from build123d import *

# Parameters (mm, degrees)
F10_DEPTH = 2
F11_DEPTH = 2
F12_DEPTH = 2
F13_DEPTH = 2
F14_W     = 8.485019207
F14_H     = 5.5162683129
F15_DEPTH = 25.4
F16_W     = 22.2342889756
F16_H     = 4.6487008221
F17_DEPTH = 25.4
F18_W     = 7.9449899495
F18_H     = 7.2886322159
F19_DEPTH = 25.4
F20_W     = 5.9225577861
F20_H     = 11.3939000294
F21_DEPTH = 25.4
F22_DEPTH = 25.4
F24_DEPTH = 10
F25_W     = 57.7732250094
F25_H     = 30.5333668366
F26_DEPTH = 25.4
F27_W     = 39.3364997581
F27_H     = 21.5767812915
F28_DEPTH = 25.4


with BuildPart() as f10:
    # F9 (on 3pt) → F10 (new body)
    with BuildSketch(Plane(origin=(3.3858576339, 10.4205982991, 0.8801059814), x_dir=(-0.9513782964, 0.3069321376, 0.0259229655), z_dir=(0.308024897, 0.9480031547, 0.0800667316))):
        Polygon((7.9863190401, -1.0910055423), (-27.9953896476, 21.7198480533), (-8.0322433603, -0.6742785071), align=None)
    extrude(amount=-F10_DEPTH)

    # F7 (on 3pt) → F11 (join)
    with BuildSketch(Plane(origin=(-2.4612159584, 1.7881780643, 4.9288143129), x_dir=(0.9052277817, 0.144920932, 0.3994503557), z_dir=(-0.4249266563, 0.3087272871, 0.8509552274))):
        Polygon((35.8818855958, -7.4339114282), (-1.9342501918, 12.1864421859), (-12.3389909213, 0), align=None)
    extrude(amount=-F11_DEPTH)

    # F6 (on 3pt) → F12 (join)
    with BuildSketch(Plane(origin=(-2.4612159584, -1.7881780643, 4.9288143129), x_dir=(0.9052277817, -0.144920932, 0.3994503557), z_dir=(-0.4249266563, -0.3087272871, 0.8509552274))):
        Polygon((-1.9342501918, -12.1864421859), (35.8818855958, 7.4339114282), (-12.3389909213, 0), align=None)
    extrude(amount=-F12_DEPTH)

    # F5 (on face) → F13 (join)
    with BuildSketch(Plane(origin=(3.3858576339, -10.4205982991, 0.8801059814), x_dir=(0.9513782964, 0.3069321376, -0.0259229655), z_dir=(0.308024897, -0.9480031547, 0.0800667316))):
        Polygon((8.0322433603, -0.6742785071), (27.9953896476, 21.7198480533), (-7.9863190401, -1.0910055423), align=None)
    extrude(amount=-F13_DEPTH)

    # F14 (on face) → F15 (cut)
    with BuildSketch(Plane(origin=(3.3858576339, -10.4205982991, 0.8801059814), x_dir=(0.9513782964, 0.3069321376, -0.0259229655), z_dir=(0.308024897, -0.9480031547, 0.0800667316))):
        with Locations((25.7894098759, 19.5572990924)):
            Rectangle(F14_W, F14_H)
    extrude(amount=F15_DEPTH, mode=Mode.SUBTRACT)

    # F16 (on face) → F17 (cut)
    with BuildSketch(Plane(origin=(-2.4612159584, 1.7881780643, 4.9288143129), x_dir=(0.9052277817, 0.144920932, 0.3994503557), z_dir=(-0.4249266563, 0.3087272871, 0.8509552274))):
        with Locations((32.4524613097, -6.6612462979)):
            Rectangle(F16_W, F16_H)
    extrude(amount=F17_DEPTH, mode=Mode.SUBTRACT)

    # F18 (on face) → F19 (cut)
    with BuildSketch(Plane(origin=(-2.4612159584, -1.7881780643, 4.9288143129), x_dir=(0.9052277817, -0.144920932, 0.3994503557), z_dir=(-0.4249266563, -0.3087272871, 0.8509552274))):
        with Locations((35.5167929083, 5.7378442725)):
            Rectangle(F18_W, F18_H)
    extrude(amount=F19_DEPTH, mode=Mode.SUBTRACT)

    # F20 (on face) → F21 (cut)
    with BuildSketch(Plane(origin=(3.3858576339, 10.4205982991, 0.8801059814), x_dir=(-0.9513782964, 0.3069321376, 0.0259229655), z_dir=(0.308024897, 0.9480031547, 0.0800667316))):
        with Locations((-26.7476057634, 18.5779468156)):
            Rectangle(F20_W, F20_H)
    extrude(amount=F21_DEPTH, mode=Mode.SUBTRACT)

    # F0 (on Top) → F22 (cut)
    with BuildSketch(Plane.XY):
        Polygon((11.027559638, -8.0119910571), (11.027559638, 8.0119910571), (-4.2121529688, 12.963673848), (-13.6308133385, 0), (-4.2121529688, -12.963673848), align=None)
    extrude(amount=-F22_DEPTH, mode=Mode.SUBTRACT)

    # F23 (on face) → F24 (join)
    with BuildSketch(Plane(origin=(0, 0, 0), x_dir=(1, 0, 0), z_dir=(0, 0, -1))):
        Polygon((6.725183616, -3.5935375892), (1.1445587857, 0), (-5.7149456211, -4.4170478538), (-1.6444061956, -10.0196647256), (6.725183616, -7.3002201464), align=None)
        Polygon((-1.6444061956, 10.0196647256), (-5.7149456211, 4.4170478538), (1.1445587857, 0), (6.725183616, 3.5935375892), (6.725183616, 7.3002201464), align=None)
        Polygon((6.725183616, 3.5935375892), (1.1445587857, 0), (6.725183616, -3.5935375892), align=None)
        Polygon((6.725183616, 7.3002201464), (6.725183616, 3.5935375892), (10.5510387165, 6.0571244693), align=None)
        Polygon((6.725183616, 3.5935375892), (6.725183616, -3.5935375892), (10.5510387165, -6.0571244693), (10.5510387165, 6.0571244693), align=None)
        Polygon((10.5510387165, -6.0571244693), (6.725183616, -3.5935375892), (6.725183616, -7.3002201464), align=None)
    extrude(amount=-F24_DEPTH)

    # F25 (on face) → F26 (cut)
    with BuildSketch(Plane(origin=(-2.4612159584, 1.7881780643, 4.9288143129), x_dir=(0.9052277817, 0.144920932, 0.3994503557), z_dir=(-0.4249266563, 0.3087272871, 0.8509552274))):
        with Locations((7.6596103609, -0.1687561162)):
            Rectangle(F25_W, F25_H)
    extrude(amount=F26_DEPTH, mode=Mode.SUBTRACT)

    # F27 (on face) → F28 (cut)
    with BuildSketch(Plane(origin=(-2.4612159584, -1.7881780643, 4.9288143129), x_dir=(0.9052277817, -0.144920932, 0.3994503557), z_dir=(-0.4249266563, -0.3087272871, 0.8509552274))):
        with Locations((5.8207563125, -4.5227890369)):
            Rectangle(F27_W, F27_H)
    extrude(amount=F28_DEPTH, mode=Mode.SUBTRACT)


solid = f10.part
CAD build for the part. Positions are in the model's coordinates, mm. A direction names the side the tool comes from. Give positions to 0.01 mm unless a question says otherwise; leave off trailing zeros. Order: outer loops, then holes, each group sorted by start corner. A loop starts at its lowest first (then second) coordinate and runs counter-clockwise, first axis right, second up. Notation, with made-up numbers: (62.5, 64) - (78.5, 64) arc R12 cw to (78.5, 79) - close; hole circle Ø9 at (56, 89). An arc over 180 degrees is marked (long way). Write each question's results on one line, items separated by ' | '.
1. Saw through at C-C on y = -8.75. List the corners of the cut face in (x, z), and give its area (3 significant figures).
Calculated:
outline: (-7.27, 0) - (8.76, 0) - (6.91, 7.08) - close | area: 56.8 mm2
2. Probe L1, parallel to X at y = -2, z = 1; L2, parallel to X at y = -5, z = 2.25; L3, parallel to Z at x = 1, y = 2. List the from-to ranges inside material, lowest first. Write a range as from..to.
Calculated:
L1: x = -10.18..-5.47, -1.96..10.55 | L2: x = -5.49..10.55 | L3: z = 0..6.58
3. 3-axis set-ups, long thin cutter, end or side, ignore diameter. For faces 1 (the face through (26.731, 0.565, 17.6)), 2 (the face through (-5.08, 1.19, 1.49)), 3 (the face through (28.82, 0.42, 19.75)): which of +Z, -Z, +X, -X, +Y, -Y reach the whole face in a straight line?
Calculated:
face 1: -Z, +X | face 2: -Z | face 3: +Y
4. Saw through at D-D on x = -8. List the corners of the cut face in (y, z).
Calculated:
outline: (-7.75, 0) - (-1.27, 0) - (0, 0.46) - (1.27, 0) - (7.75, 0) - (0, 2.81) - close
5. Saw through at B-B on x = 19. List the corners of the cut face in (y, z), and give its area (3 significant figures).
Calculated:
outline: (-4.65, 9.15) - (-2.49, 9.7) - (-2.2, 13.15) - (0, 13.94) - (2.2, 13.15) - (2.49, 9.7) - (4.65, 9.15) - (4.17, 14.78) - (0, 16.29) - (-4.17, 14.78) - close | area: 34.1 mm2
6. Pin check, flat tips, straight feed: pin 1 (1 mm diameter, centred on y = 8, z = 4.5, fed in from -X); pin 2 (8 mm diameter, centred on x = 19, z = 3.5, fed in from +Y); pin 3 (3 mm diameter, centred on x = 5, y = -6.5, fed in from +Z); pin 4 (1.5 mm diameter, centred on x = 8, z = 12, fed in from +Y). Stop position of each tip, or through.
Calculated:
pin 1: stops at x = 0.13 | pin 2: stops at y = 6.24 | pin 3: stops at z = 7.87 | pin 4: passes through
7. Pull direction X, two halves, no side cores. Call faces 4 (the face through (17.98, -4.02, 8.25)), 5 (the face through (4.859, 4.554, 7.581)), 6 (the face through (-1.48, 1.69, 1.92)): released by +X, released by -X, zero draft, split by the parting line, or undercut.
Calculated:
face 4: released by +X | face 5: released by -X | face 6: undercut
8. Saw through at A-A on z = 12.25. List the corners of the cut face in (x, y).
Calculated:
outline: (10.9, 0) - (15.03, -5.68) - (21.7, -3.51) - (21.22, -1.55) - (17.59, -2.73) - (15.61, 0) - (17.59, 2.73) - (21.22, 1.55) - (21.7, 3.51) - (15.03, 5.68) - close
